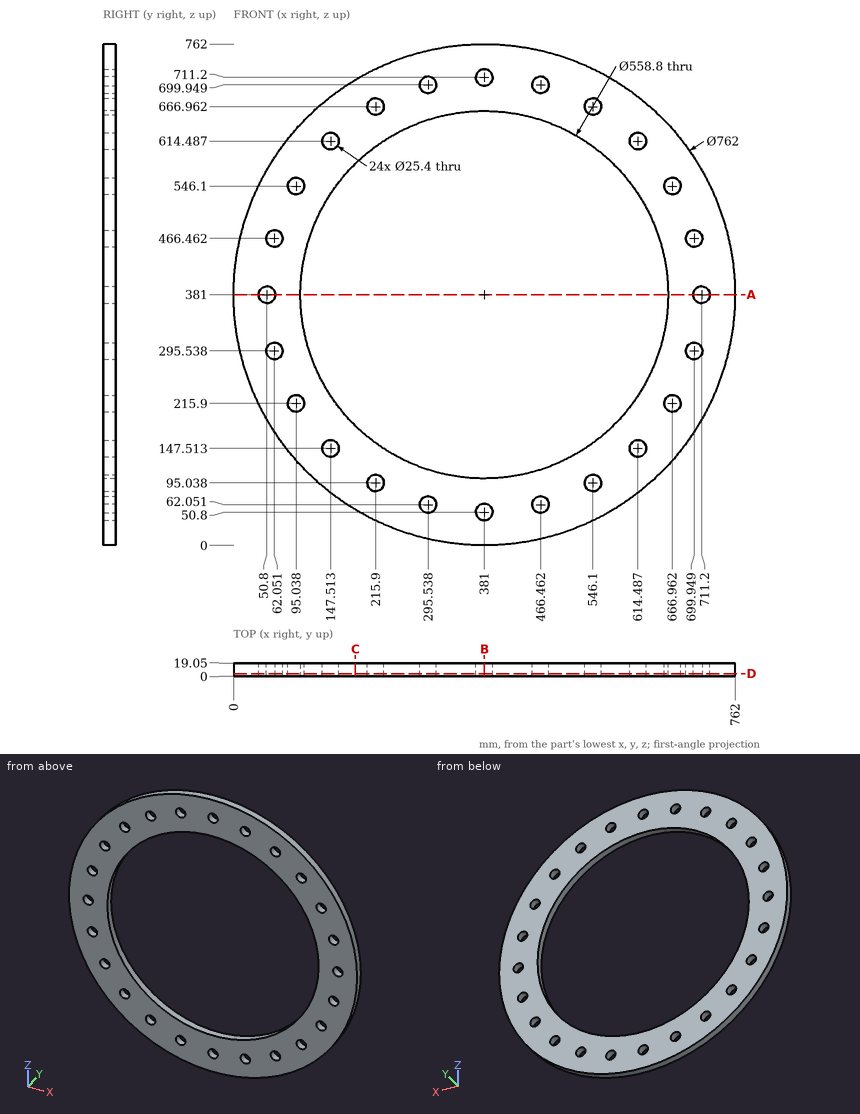
Part print with two shaded views. Sizes in mm from the minimum x, y, z corner. Round coordinates to 2 decimals unless told otherwise and drop trailing zeros. Loops run counter-clockwise (first coordinate to the right, second up) from the corner with the lowest first, then second, coordinate; pieces in that order, holes last. Notation, with made-up numbers: M 51,69.25 L 91,69.25 A25 ccw 91,82.25 Z; hole C 25.25,45.25 d7. An arc over 180 degrees is marked long. Put each result on its own line as item: value. Start each with the question number.
Item 1: Cut at A-A (z = 381). List the corners of the cut face in (x, y), then the cut area to 3 significant figures.
Item 2: Drop flat-ended pins along their axis: P1, Ø20.5, axis at x = 466.46, z = 62.05, coming from the -Y side; P2, Ø5, axis at x = 256.5, y = 11.5, coming from the +Z side; P3, Ø1.5, axis at y = 2, z = 566.5, coming from the -X side; P4, Ø4, axis at x = 133.5, y = 13.5, coming from the +Z side. Give the stop position or say it passes through.
Item 3: Cut at D-D (y = 3.75). Give the number of separate pieces and of enclosed holes in the cut face, then the cut area to 3 significant figures.
Item 4: Drill centre lines: line 1 along Z through (x, y) = (152, 9.75) (1 decimal); line 2 along X through (y, z) = (9.5, 215.9); line 3 along X through (y, z) = (10.25, 605.5) (1 decimal). Where is each one in solid material? Low to high.
Item 5: Cut at B-B (x = 381). List the corners of the cut face in (y, z), then the cut area to 3 significant figures.
Item 6: Cut at C-C (x = 185). List the corners of the cut face in (y, z), then the cut area to 3 significant figures.
Answer block:
1. outline: M 0,0 L 38.1,0 L 38.1,19.05 L 0,19.05 Z; M 63.5,0 L 101.6,0 L 101.6,19.05 L 63.5,19.05 Z; M 660.4,0 L 698.5,0 L 698.5,19.05 L 660.4,19.05 Z; M 723.9,0 L 762,0 L 762,19.05 L 723.9,19.05 Z
1. area: 2,900 mm2
2. P1: through
2. P2: z = 741.94
2. P3: x = 47.79
2. P4: z = 672.36
3. separate pieces: 1
3. enclosed holes: 25
3. area: 199,000 mm2
4. line 1: 76.5 to 135.6, 159.4 to 220.9, 541.1 to 602.6, 626.4 to 685.5
4. line 2: 37.63 to 82.34, 107.74 to 155.6, 606.4 to 654.26, 679.66 to 724.37
4. line 3: 73.2 to 138.5, 156.5 to 214.7, 547.3 to 605.5, 623.5 to 688.8
5. outline: M 0,0 L 19.05,0 L 19.05,38.1 L 0,38.1 Z; M 0,63.5 L 19.05,63.5 L 19.05,101.6 L 0,101.6 Z; M 0,660.4 L 19.05,660.4 L 19.05,698.5 L 0,698.5 Z; M 0,723.9 L 19.05,723.9 L 19.05,762 L 0,762 Z
5. area: 2,900 mm2
6. outline: M 0,54.28 L 19.05,54.28 L 19.05,181.88 L 0,181.88 Z; M 0,580.12 L 19.05,580.12 L 19.05,707.72 L 0,707.72 Z
6. area: 4,860 mm2
